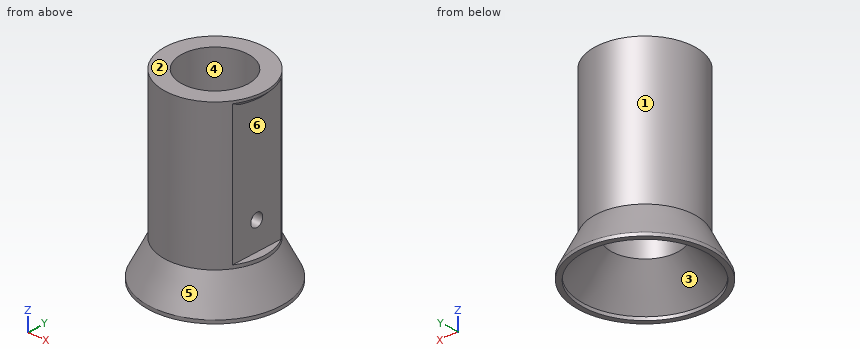
Autodesk Inventor part; units mm, degrees
ref_plane "YZ Plane" through (0, 0, 0) normal (1, 0, 0) x (0, 1, 0)
ref_plane "XZ Plane" through (0, 0, 0) normal (0, 1, 0) x (-1, 0, 0)
ref_plane "XY Plane" through (0, 0, 0) normal (0, 0, 1) x (1, 0, 0)
sketch "Sketch1" plane through (0, 0, 0) normal (0, 0, 1) x (1, 0, 0)
  circle A0 centre (0, 0) radius 23.495
  circle A1 centre (0, 0) radius 25.4
  dimension "d4" = 46.99
  dimension "d5" = 50.8
extrude "Extrusion1" add sketch "Sketch1" along normal blind 1.27
ref_plane "Work Plane1" through (0, 0, 13.97) normal (0, 0, 1) x (1, 0, 0)
sketch "Sketch2" plane through (0, 0, 13.97) normal (0, 0, 1) x (1, 0, 0)
  circle A0 centre (0, 0) radius 19.05
  circle A1 centre (0, 0) radius 12.7
  dimension "d9" = 38.1
  dimension "d10" = 25.4
sketch "Sketch3" plane through (0, 0, 13.97) normal (0, 0, 1) x (1, 0, 0)
  circle A0 centre (0, 0) radius 10.795
  line L0 (0, 10.795) -> (0, 7.0011) construction
ref_plane "Work Plane2" through (0, 10.795, 13.97) normal (1, 0, 0) x (0, -1, 0)
ref_plane "Work Plane3" through (0, 0, 15.24) normal (0, 0, 1) x (1, 0, 0)
sketch "Sketch5" plane through (0, 0, 15.24) normal (0, 0, 1) x (1, 0, 0)
  circle A0 centre (0, 0) radius 12.7
  circle A1 centre (0, 0) radius 19.05
  dimension "d20" = 38.1
  dimension "d21" = 25.4
extrude "Extrusion3" add sketch "Sketch5" along normal blind 50.8
sketch "Sketch6" plane through (0, 10.795, 13.97) normal (1, 0, 0) x (0, -1, 0)
  point P0 (10.795, 13.97)
extrude "Extrusion4" add sketch "Sketch2" along normal blind 1.27
sketch "Sketch7" plane through (0, 10.795, 13.97) normal (1, 0, 0) x (0, -1, 0)
  line L0 (-14.605, 12.7) -> (36.195, 12.7)
  line L1 (29.845, 0) -> (-8.255, 0)
  line L2 (-14.605, 12.7) -> (-8.255, 0)
  line L3 (-1.905, 0) -> (23.495, 0)
  line L4 (-8.255, 0) -> (-1.905, 0)
  line L5 (34.29, 12.7) -> (-12.7, 12.7)
  line L6 (-1.905, 0) -> (-12.7, 12.7)
  line L7 (-12.7, 12.7) -> (-14.605, 12.7)
  line L8 (10.795, 0) -> (10.795, 4.3567) construction
  point P0 (10.795, 13.97)
revolve "Revolution2" add sketch "Sketch7" angle 360 about axis through (0, 0, 13.97) along (0, 0, -1)
sketch "Sketch8" plane through (0, 10.795, 13.97) normal (1, 0, 0) x (0, -1, 0)
  point P0 (10.795, 13.97)
sketch "Sketch9" plane through (0, 0, 66.04) normal (0, 0, 1) x (1, 0, 0)
  circle A0 centre (0, 0) radius 19.05
  line L0 (16.0969, 10.1879) -> (16.0969, -10.1879)
  arc A1 (16.0969, -10.1879) -> (16.0969, 10.1879) centre (0, 0) ccw
extrude "Extrusion5" cut sketch "Sketch9" against normal blind 50.8 contours A0 L0 picked at (16.6372, -2.3328)
sketch "Sketch10" plane through (16.0969, -10.1879, 66.04) normal (1, 0, 0) x (0, 0, -1)
  circle A0 centre (40.3701, 10.1879) radius 2.5
  point P0 (66.04, 10.1879)
  dimension "d24" = 5
extrude "Extrusion6" cut sketch "Sketch10" against normal blind 12.7
sketch "Sketch11" plane through (0, 0, 66.04) normal (0, 0, 1) x (1, 0, 0)
  circle A0 centre (0, 0) radius 19.05
  circle A1 centre (0, 0) radius 12.7
extrude "Extrusion7" add sketch "Sketch11" along normal blind 2.54
chamfer "Chamfer1" distance 1.5875 angle 45 2 edges at (18.2968, 5.3036, 66.04) (18.2968, -5.3036, 66.04)
properties part number "uvlight holder"
Read the model definition and answer for the solid it produces. Units are mm, in the model's axes. Face numbers are marked on the shaded views. A direction names the side the tool comes from. Give positions to 0.01 mm unless a question says otherwise; leave off trailing zeros. Order: outer loops, then holes, each group sorted by start corner. A loop starts at its lowest first (then second) coordinate and runs counter-clockwise, first axis right, second up. Notation, with made-up numbers: (-17, 53.5) -> (-1, 53.5) arc R15 ccw to (-1, 65.5) -> close; hole circle Ø6 at (15, 35). An arc over 180 degrees is marked (long way). One line per item, written item: value. Start each with the question number.
(1) The part is cut by section D-D (z = 36). Determine the outline of the cut face in (x, y).
(2) The part is cut by section C-C (z = 9). Determine the outline of the cut face in (x, y) (1 decimal), and give its area (3 significant figures).
(3) For a pull along Y with two mould halves and no side action, classify the marked faces 3, 4, 5 and 6 as released by +Y, released by -Y, zero draft, split by the parting line, or undercut.
(4) A tool of negligible diameter and unlimited length cuts with its end or side. For the marked faces 1 and 2, from which of +Z, -Z, +X, -X, +Y, -Y can it reach the whole face along a straight path? Write none if from no direction.
(5) Flat-ended cylindrical pins translate along their axes: P1, Ø2, axis at y = 13, z = 10.5, coming from the -X side; P2, Ø12, axis at x = -7.5, y = 11, coming from the -Z side; P3, Ø6, axis at y = 0.5, z = 18, coming from the -X side. Find the tip coordinate at first contact, or state that the pin passes through.
(6) The part is cut by section B-B (x = 0). Determine the outline of the cut face in (y, z) (3 decimals), and give its area (3 significant figures).
(7) Straight lines are drawn through the part: L1, parallel to Y at x = 0, z = 1.05 (3 decimals); L2, parallel to Y at x = 0, z = 48. For each, find the intervals that lie inside material, in ascending order.
(8) The part is cut by section A-A (y = 0). State how many separate pieces and enclosed holes the cut face has, and give its area (3 significant figures).
Taken from the geometry:
1. outline: (16.1, -10.19) -> (16.1, 10.19) arc R19.05 ccw (long way) to start; hole circle Ø25.4 at (0, 0)
2. outline: circle Ø43.1 at (0, 0); hole circle Ø33.8 at (0, 0)
2. area: 557 mm^2
3. face 3: undercut
3. face 4: undercut
3. face 5: split by the parting line
3. face 6: zero draft
4. face 1: +Z
4. face 2: +Z, +X, -X, +Y, -Y
5. P1: x = -17.2
5. P2: z = 6.19
5. P3: x = -19.05
6. outline: (-25.4, 0) -> (-23.495, 0) -> (-23.495, 1.27) -> (-12.7, 13.97) -> (-12.7, 68.58) -> (-19.05, 68.58) -> (-19.05, 13.97) -> (-25.4, 1.27) -> close; (12.7, 13.97) -> (23.495, 1.27) -> (23.495, 0) -> (25.4, 0) -> (25.4, 1.27) -> (19.05, 13.97) -> (19.05, 68.58) -> (12.7, 68.58) -> close
6. area: 803 mm^2
7. L1: -25.4 to -23.495, 23.495 to 25.4
7. L2: -19.05 to -12.7, 12.7 to 19.05
8. separate pieces: 3
8. enclosed holes: 0
8. area: 635 mm^2
